Job drawing, mm, ordinate dimensions from the low corner. One solid piece. A direction names the side the tool comes from. Give positions to 0.01 mm unless a question says otherwise; leave off trailing zeros. Loops run counter-clockwise (first coordinate to the right, second up) from the corner with the lowest first, then second, coordinate; pieces in that order, holes last. Notation, with made-up numbers: M -0.5,13.25 L 22.5,13.25 A10 cw 22.5,29.25 Z; hole C 23.5,20 d8. An arc over 180 degrees is marked long. One line per question, with ' | ' between items.
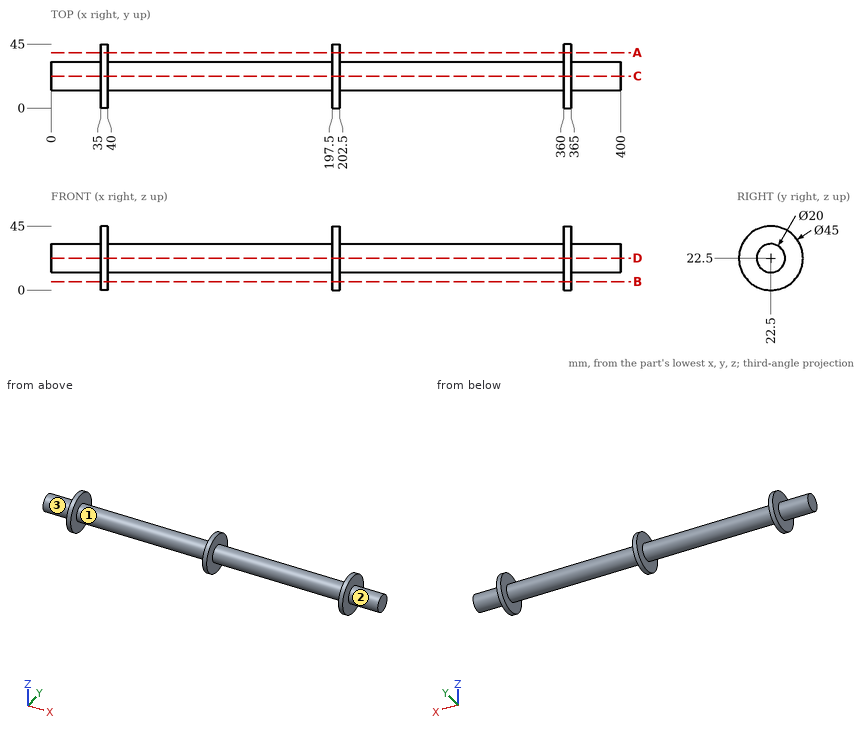
Item 1: Drop flat-ended pins along their axis: P1, Ø8, axis at y = 36, z = 12.5, coming from the -X side; P2, Ø8, axis at y = 5.5, z = 25, coming from the +X side; P3, Ø1.5, axis at x = 356.5, z = 28.5, coming from the +Y side. Give the stop position or say it passes through.
Conclusion:
P1: x = 35 | P2: x = 365 | P3: y = 31.01
Item 2: Saw through at A-A on y = 39. Give the cut face in (x, z).
Conclusion:
outline: M 35,7.2 L 40,7.2 L 40,37.8 L 35,37.8 Z; M 197.5,7.2 L 202.5,7.2 L 202.5,37.8 L 197.5,37.8 Z; M 360,7.2 L 365,7.2 L 365,37.8 L 360,37.8 Z
Item 3: Drill centre lines: line 1 along X through (y, z) = (35.5, 34); line 2 along Z through (x, y) = (205, 22.5); line 3 along Y through (x, z) = (380, 30). Where is each one in solid material? Low to high. Write a range as [from, to].
Conclusion:
line 1: [35, 40], [197.5, 202.5], [360, 365] | line 2: [12.5, 32.5] | line 3: [15.89, 29.11]
Item 4: Saw through at C-C on y = 22.5. Give the cut face in (x, z), and give its area (4 significant figures).
Conclusion:
outline: M 0,12.5 L 35,12.5 L 35,0 L 40,0 L 40,12.5 L 197.5,12.5 L 197.5,0 L 202.5,0 L 202.5,12.5 L 360,12.5 L 360,0 L 365,0 L 365,12.5 L 400,12.5 L 400,32.5 L 365,32.5 L 365,45 L 360,45 L 360,32.5 L 202.5,32.5 L 202.5,45 L 197.5,45 L 197.5,32.5 L 40,32.5 L 40,45 L 35,45 L 35,32.5 L 0,32.5 Z | area: 8,375 mm²
Item 5: 3-axis set-ups, long thin cutter, end or side, ignore diameter. For the marked faces 1, 2 and 3: which of +Z, -Z, +X, -X, +Y, -Y reach the whole face in a straight line?
Conclusion:
face 1: none | face 2: +X | face 3: -X
